Check sheet for the modelled part. Datum: model origin and axes. Units: mm. Give positions to 0.01 mm unless a question says otherwise; leave off trailing zeros. Loops run counter-clockwise (first coordinate to the right, second up) from the corner with the lowest first, then second, coordinate; pieces in that order, holes last. Notation, with made-up numbers: (-34, -1) - (16, -1) arc R4 ccw to (16, 6) - close; hole circle Ø7 at (77, 9). An arc over 180 degrees is marked (long way). Answer in a Markdown table with one row per item. Add a question column.
(1) Sectioned sample at B-B on z = 0. Enter the section's corners in (x, y) (3 decimals), then the cut area to 3 significant figures.
(2) Go/stop test with flat-tipped pins: P1, Ø5, axis at x = 22.86, z = -9.652, coming from the -Y side; P2, Ø1, axis at y = 1.5, z = -18.5, coming from the +X side; P3, Ø1.5, axis at y = 3.5, z = -2.5, coming from the +X side; P4, Ø2, axis at y = 3, z = 0.5, coming from the +X side. Record where each tip stops, or that it passes through.
(3) Sectioned sample at C-C on y = 2.4. Enter the section's corners in (x, z) (3 decimals).
(4) Sectioned sample at D-D on x = 18.5. Enter the section's corners in (y, z) (1 decimal), then the cut area to 3 significant figures.
(5) Sectioned sample at A-A on x = 0. Enter the section's corners in (y, z) (3 decimals).
(6) Thickness scan on L1, parallel to X at y = 2.4, z = -2; L2, parallel to Z at x = 22.86, y = 3; L3, parallel to X at y = 1.3, z = 8. Record the ranges inside material, lowest first.
from build123d import *

# Parameters (mm, degrees)
SKETCH2_R           = 2.706768225
SKETCH2_W           = 21.082
SKETCH2_H           = 21.082
BOSS_EXTRUDE1_DEPTH = 4.445
FILLET1_R           = 3.175
FILLET2_R           = 1.016
CHAMFER1_SIZE       = 0.508


with BuildPart() as part:
    # Sketch2 → Boss-Extrude1 (new body)
    with BuildSketch(Plane(origin=(0, 0, 0), x_dir=(1, 0, 0), z_dir=(0, 1, 0))):
        with BuildLine():
            Line((11.504506555, 42.935402979), (5.259202996, 19.62761279))
            ThreePointArc((5.259202996, 19.62761279), (-14.368409794, -14.368409794), (19.62761279, 5.259202996))
            Line((19.62761279, 5.259202996), (42.935402979, 11.504506555))
            ThreePointArc((42.935402979, 11.504506555), (31.430896424, 31.430896424), (11.504506555, 42.935402979))
        make_face()
        with Locations((22.86, 9.652)):
            Circle(SKETCH2_R, mode=Mode.SUBTRACT)
        Rectangle(SKETCH2_W, SKETCH2_H, mode=Mode.SUBTRACT)
    extrude(amount=BOSS_EXTRUDE1_DEPTH)

    # Fillet1
    fillet1_edges = [part.edges().sort_by_distance(p)[0] for p in [
        (42.935402979, 2.2225, -11.504506555),
        (19.62761279, 2.2225, -5.259202996),
        (5.259202996, 2.2225, -19.62761279),
        (11.504506555, 2.2225, -42.935402979),
    ]]
    fillet(fillet1_edges, radius=FILLET1_R)

    # Fillet2
    fillet2_edges = [part.edges().sort_by_distance(p)[0] for p in [
        (10.541, 2.2225, 10.541),
        (10.541, 2.2225, -10.541),
        (-10.541, 2.2225, -10.541),
        (-10.541, 2.2225, 10.541),
    ]]
    fillet(fillet2_edges, radius=FILLET2_R)

    # Chamfer1
    chamfer1_edges = [part.edges().sort_by_distance(p)[0] for p in [
        (20.153231775, 0, -9.652),
        (20.153231775, 4.445, -9.652),
    ]]
    chamfer(chamfer1_edges, length=CHAMFER1_SIZE)


solid = part.part
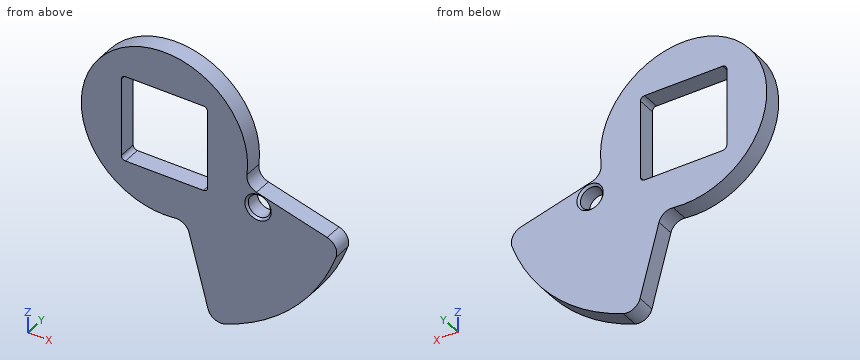
Reply:
| question | item | result |
|---|---|---|
| 1 | outline | (-20.32, 0) - (-10.541, 0) - (-10.541, 4.445) - (-20.32, 4.445) - close; (10.541, 0) - (20.32, 0) - (20.32, 4.445) - (10.541, 4.445) - close |
| 1 | area | 86.9 mm^2 |
| 2 | P1 | through |
| 2 | P2 | x = 40.64 |
| 2 | P3 | x = 20.24 |
| 2 | P4 | x = 20.32 |
| 3 | outline | (2.559, -20.158) arc R3.175 cw to (6.025, -22.486) - (10.651, -39.75) arc R3.175 ccw to (14.773, -41.923) arc R44.45 ccw to (41.923, -14.773) arc R3.175 ccw to (39.75, -10.651) - (22.486, -6.025) arc R3.175 cw to (20.158, -2.559) arc R20.32 ccw (long way) to start; hole (-10.541, -9.525) arc R1.016 ccw to (-9.525, -10.541) - (9.525, -10.541) arc R1.016 ccw to (10.541, -9.525) - (10.541, 9.525) arc R1.016 ccw to (9.525, 10.541) - (-9.525, 10.541) arc R1.016 ccw to (-10.541, 9.525) - close; hole circle Ø5.414 at (22.86, -9.652) |
| 4 | outline | (0, -40.4) - (4.4, -40.4) - (4.4, 8.4) - (0, 8.4) - close |
| 4 | area | 217 mm^2 |
| 5 | outline | (0, -20.32) - (4.445, -20.32) - (4.445, -10.541) - (0, -10.541) - close; (0, 10.541) - (4.445, 10.541) - (4.445, 20.32) - (0, 20.32) - close |
| 6 | L1 | -20.22 to -10.54, 10.54 to 20.22 |
| 6 | L2 | -38.12 to -12.36, -6.95 to -6.13 |
| 6 | L3 | -18.68 to -10.54, 10.54 to 18.68 |
